```python
from build123d import *

# Parameters (mm, degrees)
SKETCH1_W               = 279.4
SKETCH1_H               = 76.2
BOSS_EXTRUDE1_DEPTH     = 3
SKETCH3_W               = 3
SKETCH3_H               = 7.8
CUT_EXTRUDE1_DEPTH      = 145.833352512
LPATTERN1_COUNT         = 4
LPATTERN1_PITCH         = 22.8
MIRROR1_COPY_1_SKETCH_W = 3
MIRROR1_COPY_1_SKETCH_H = 7.8
MIRROR1_COPY_1_DEPTH    = 145.833352512
MIRROR1_COPY_2_SKETCH_W = 3
MIRROR1_COPY_2_SKETCH_H = 7.8
MIRROR1_COPY_2_DEPTH    = 145.833352512
MIRROR1_COPY_3_SKETCH_W = 3
MIRROR1_COPY_3_SKETCH_H = 7.8
MIRROR1_COPY_3_DEPTH    = 145.833352512
SKETCH4_W               = 3
SKETCH4_H               = 15
CUT_EXTRUDE2_DEPTH      = 10
LPATTERN2_COUNT         = 3
LPATTERN2_PITCH         = 22.8
MIRROR2_COPY_1_SKETCH_W = 3
MIRROR2_COPY_1_SKETCH_H = 15
MIRROR2_COPY_1_DEPTH    = 10
MIRROR2_COPY_2_SKETCH_W = 3
MIRROR2_COPY_2_SKETCH_H = 15
MIRROR2_COPY_2_DEPTH    = 10
SKETCH5_W               = 3
SKETCH5_H               = 7.8
BOSS_EXTRUDE2_DEPTH     = 3
LPATTERN3_COUNT         = 8
LPATTERN3_PITCH         = 22.8
F_6_CLEARANCE_HOLE1_D   = 3.7973
F_6_CLEARANCE_HOLE2_D   = 3.7973
CUT_EXTRUDE3_REACH      = 147.651
SKETCH10_W              = 20.2
SKETCH10_H              = 6.7
F_6_CLEARANCE_HOLE3_D   = 3.7973


with BuildPart() as part:
    # Sketch1 → Boss-Extrude1 (new body)
    with BuildSketch(Plane(origin=(0, 0, 0), x_dir=(0, 0, -1), z_dir=(1, 0, 0))):
        Rectangle(SKETCH1_W, SKETCH1_H)
    extrude(amount=-BOSS_EXTRUDE1_DEPTH)

    # Sketch3 → Cut-Extrude1 (cut, through all)
    with BuildSketch(Plane.ZY.offset(3)):
        with Locations((-138.2, 34.2)):
            Rectangle(SKETCH3_W, SKETCH3_H)
    cut_extrude1 = extrude(amount=-CUT_EXTRUDE1_DEPTH, mode=Mode.SUBTRACT)

    # LPattern1: Cut-Extrude1 ×4
    with Locations(*[(0, -i * LPATTERN1_PITCH, 0) for i in range(1, LPATTERN1_COUNT)]):
        add(cut_extrude1, mode=Mode.SUBTRACT)

    # Mirror1: Cut-Extrude1 across plane
    add(cut_extrude1.mirror(Plane.XY), mode=Mode.SUBTRACT)

    # Mirror1 copy 1 sketch → Mirror1 copy 1 (cut, through all)
    with BuildSketch(Plane(origin=(-3, -22.8, 0), x_dir=(0, 0, -1), z_dir=(-1, 0, 0))):
        with Locations((-138.2, -34.2)):
            Rectangle(MIRROR1_COPY_1_SKETCH_W, MIRROR1_COPY_1_SKETCH_H)
    extrude(amount=-MIRROR1_COPY_1_DEPTH, mode=Mode.SUBTRACT)

    # Mirror1 copy 2 sketch → Mirror1 copy 2 (cut, through all)
    with BuildSketch(Plane(origin=(-3, -45.6, 0), x_dir=(0, 0, -1), z_dir=(-1, 0, 0))):
        with Locations((-138.2, -34.2)):
            Rectangle(MIRROR1_COPY_2_SKETCH_W, MIRROR1_COPY_2_SKETCH_H)
    extrude(amount=-MIRROR1_COPY_2_DEPTH, mode=Mode.SUBTRACT)

    # Mirror1 copy 3 sketch → Mirror1 copy 3 (cut, through all)
    with BuildSketch(Plane(origin=(-3, -68.4, 0), x_dir=(0, 0, -1), z_dir=(-1, 0, 0))):
        with Locations((-138.2, -34.2)):
            Rectangle(MIRROR1_COPY_3_SKETCH_W, MIRROR1_COPY_3_SKETCH_H)
    extrude(amount=-MIRROR1_COPY_3_DEPTH, mode=Mode.SUBTRACT)

    # Sketch4 → Cut-Extrude2 (cut)
    with BuildSketch(Plane(origin=(0, 0, 0), x_dir=(0, 0, -1), z_dir=(1, 0, 0))):
        with Locations((-95.2, 22.8)):
            Rectangle(SKETCH4_W, SKETCH4_H)
    cut_extrude2 = extrude(amount=-CUT_EXTRUDE2_DEPTH, mode=Mode.SUBTRACT)

    # LPattern2: Cut-Extrude2 ×3
    with Locations(*[(0, -i * LPATTERN2_PITCH, 0) for i in range(1, LPATTERN2_COUNT)]):
        add(cut_extrude2, mode=Mode.SUBTRACT)

    # Mirror2: Cut-Extrude2 across plane
    add(cut_extrude2.mirror(Plane.XY), mode=Mode.SUBTRACT)

    # Mirror2 copy 1 sketch → Mirror2 copy 1 (cut)
    with BuildSketch(Plane(origin=(0, -22.8, 0), x_dir=(0, 0, 1), z_dir=(1, 0, 0))):
        with Locations((-95.2, -22.8)):
            Rectangle(MIRROR2_COPY_1_SKETCH_W, MIRROR2_COPY_1_SKETCH_H)
    extrude(amount=-MIRROR2_COPY_1_DEPTH, mode=Mode.SUBTRACT)

    # Mirror2 copy 2 sketch → Mirror2 copy 2 (cut)
    with BuildSketch(Plane(origin=(0, -45.6, 0), x_dir=(0, 0, 1), z_dir=(1, 0, 0))):
        with Locations((-95.2, -22.8)):
            Rectangle(MIRROR2_COPY_2_SKETCH_W, MIRROR2_COPY_2_SKETCH_H)
    extrude(amount=-MIRROR2_COPY_2_DEPTH, mode=Mode.SUBTRACT)

    # Sketch5 → Boss-Extrude2 (add)
    with BuildSketch(Plane(origin=(0, 38.1, 0), x_dir=(1, 0, 0), z_dir=(0, 1, 0))):
        with Locations((-1.5, -79.8)):
            Rectangle(SKETCH5_W, SKETCH5_H)
    boss_extrude2 = extrude(amount=BOSS_EXTRUDE2_DEPTH)

    # LPattern3: Boss-Extrude2 ×8
    with Locations(*[(0, 0, -i * LPATTERN3_PITCH) for i in range(1, LPATTERN3_COUNT)]):
        add(boss_extrude2)

    # #6 Clearance Hole1 (through all)
    with Locations(Plane.ZY.offset(3)):
        with Locations((-28.9, -11.55), (-28.9, -26.55), (28.9, -26.55), (28.9, -11.55)):
            Hole(F_6_CLEARANCE_HOLE1_D / 2)

    # #6 Clearance Hole2 (through all)
    with Locations(Plane(origin=(0, 0, 0), x_dir=(0, 0, -1), z_dir=(1, 0, 0))):
        with Locations((-9, 0.9), (9, 0.9)):
            Hole(F_6_CLEARANCE_HOLE2_D / 2)

    # Sketch10 → Cut-Extrude3 (cut, up to next)
    with BuildSketch(Plane.ZY.offset(3), mode=Mode.PRIVATE) as cut_extrude3_sk1:
        with Locations((114.7, -15.8)):
            Rectangle(SKETCH10_W, SKETCH10_H)
    cut_extrude3_tool1 = extrude(cut_extrude3_sk1.sketch, amount=-CUT_EXTRUDE3_REACH, mode=Mode.PRIVATE) & part.part
    # Sketch10 → Cut-Extrude3 (cut, up to next)
    with BuildSketch(Plane.ZY.offset(3), mode=Mode.PRIVATE) as cut_extrude3_sk2:
        with Locations((-114.7, -15.8)):
            Rectangle(SKETCH10_W, SKETCH10_H)
    cut_extrude3_tool2 = extrude(cut_extrude3_sk2.sketch, amount=-CUT_EXTRUDE3_REACH, mode=Mode.PRIVATE) & part.part
    add(cut_extrude3_tool1.solids().sort_by_distance((-3, -15.8, 114.7))[0], mode=Mode.SUBTRACT)
    add(cut_extrude3_tool2.solids().sort_by_distance((-3, -15.8, -114.7))[0], mode=Mode.SUBTRACT)

    # #6 Clearance Hole3 (through all)
    with Locations(Plane.ZY.offset(3)):
        with Locations((-114.7, -8.45), (-114.7, -23.15), (114.7, -23.15), (114.7, -8.45)):
            Hole(F_6_CLEARANCE_HOLE3_D / 2)


solid = part.part
```
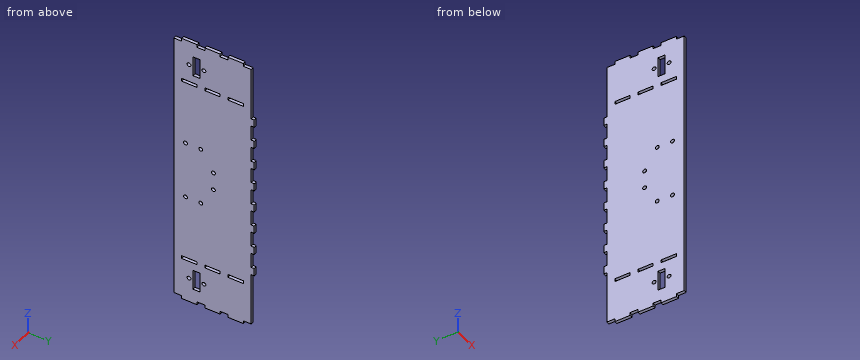
Could you check a few things on this model? Use its own coordinates, in mm. Round coordinates to 2 decimals unless told otherwise and drop trailing zeros. Loops run counter-clockwise (first coordinate to the right, second up) from the corner with the lowest first, then second, coordinate; pieces in that order, holes last. Notation, with made-up numbers: M 81,12.5 L 97,12.5 A30 cw 97,50.5 Z; hole C 67,18 d2. An arc over 180 degrees is marked long. Put each result on its own line as item: value.
Q1. Imagine slicing it at B-B (z = 90.5). Write out the boundary of the cut face in (x, y), then the cut area to 3 significant figures.
Check result:
outline: M -3,-38.1 L 0,-38.1 L 0,38.1 L -3,38.1 Z
area: 229 mm2
Q2. I need wall thicknesses on probe 1 along Y at (x, z) = (-0.95, -114.7); probe 2 along Z at (x, y) = (-1.15, -17); probe 3 along Y at (x, z) = (-0.7, -28.9). Which ranges of each line are inside material? Lowest first, please.
Check result:
probe 1: -38.1 to -25.05, -21.25 to -19.15, -12.45 to -10.35, -6.55 to 38.1
probe 2: -139.7 to -124.8, -104.6 to -96.7, -93.7 to 93.7, 96.7 to 104.6, 124.8 to 139.7
probe 3: -38.1 to -28.45, -24.65 to -13.45, -9.65 to 38.1
Q3. For pin 1 (0.9 mm diameter, centred on x = -2, y = 39, fed in from +Z); pin 2 (1.5 mm diameter, centred on x = -1, z = 46, fed in from +Y), each with a flat end and sliding along its axis, tell me the tip position at first contact or that it passes through.
Check result:
pin 1: z = 83.7
pin 2: y = 38.1
Q4. Imagine slicing it at A-A (x = -0.5). State how many separate pieces and enclosed holes the cut face has, then the cut area to 3 significant figures.
Check result:
separate pieces: 1
enclosed holes: 18
area: 20,600 mm2
